Read the model definition and answer for the solid it produces. Units are mm, in the model's axes. Coordinates: 2 decimals unless noted, no trailing zeros. Order: outer loops, then holes, each group sorted by start corner. A loop starts at its lowest first (then second) coordinate and runs counter-clockwise, first axis right, second up. Notation, with made-up numbers: M 7,-8.5 L 29,-8.5 A6 ccw 29,-0.5 Z; hole C 35.25,61.25 d10. An arc over 180 degrees is marked long. Use a Markdown table: item, result. Add a question column.
1) Find section B-B on x = 131.15. Write down the section's boundary in (y, z), plus the area to 3 significant figures.
2) Find section D-D on x = 30.5. Write down the section's boundary in (y, z), plus the area to 3 significant figures.
3) Find section C-C on y = 2. Count the separate pieces of the cut face and the enclosed holes in it, plus the area to 3 significant figures.
4) Find the intervals of material crossed by probe 1 along X at (y, z) = (4.5, -50); probe 2 along Z at (x, y) = (119, 4.25); probe 3 along Z at (x, y) = (131.15, 4.5), in increasing order. Write a range as [from, to].
5) This flat-tipped pin is pushed along its axis until it touches: pin 1 Ø2.5 at (x, z) = (8.85, -50) entering from -Y. Where does it stop, or does it pass through?
6) Find section A-A on x = 68. Write down the section's boundary in (y, z), plus the area to 3 significant figures.
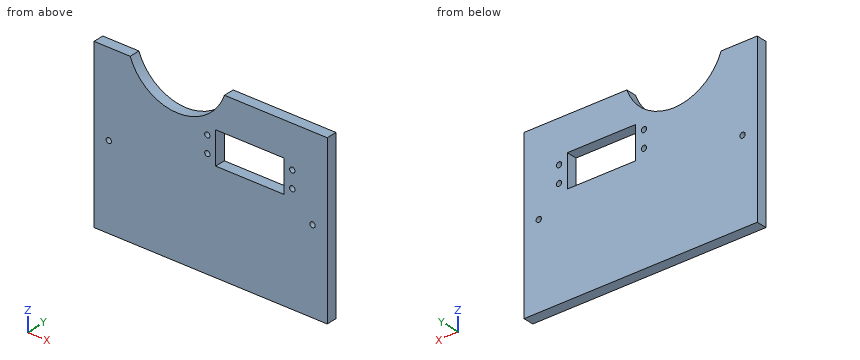
from build123d import *

# Parameters (mm, degrees)
SKETCH1_W           = 140
SKETCH1_H           = 100
BOSS_EXTRUDE1_DEPTH = 6.35
SKETCH2_W           = 41
SKETCH2_H           = 19.5
CUT_EXTRUDE1_DEPTH  = 10
SKETCH3_R           = 30
CUT_EXTRUDE2_DEPTH  = 10
SKETCH4_R           = 1.5875
CUT_EXTRUDE3_DEPTH  = 10


with BuildPart() as part:
    # Sketch1 → Boss-Extrude1 (new body)
    with BuildSketch(Plane(origin=(0, 0, 0), x_dir=(1, 0, 0), z_dir=(0, 1, 0))):
        with Locations((70, 50)):
            Rectangle(SKETCH1_W, SKETCH1_H)
    extrude(amount=BOSS_EXTRUDE1_DEPTH)

    # Sketch2 → Cut-Extrude1 (cut)
    with BuildSketch(Plane(origin=(0, 6.35, 0), x_dir=(1, 0, 0), z_dir=(0, 1, 0))):
        with Locations((93.5, 30.25)):
            Rectangle(SKETCH2_W, SKETCH2_H)
    extrude(amount=-CUT_EXTRUDE1_DEPTH, mode=Mode.SUBTRACT)

    # Sketch3 → Cut-Extrude2 (cut)
    with BuildSketch(Plane(origin=(0, 6.35, 0), x_dir=(1, 0, 0), z_dir=(0, 1, 0))):
        with Locations((50, -10)):
            Circle(SKETCH3_R)
    extrude(amount=-CUT_EXTRUDE2_DEPTH, mode=Mode.SUBTRACT)

    # Sketch4 → Cut-Extrude3 (cut)
    with BuildSketch(Plane(origin=(0, 6.35, 0), x_dir=(1, 0, 0), z_dir=(0, 1, 0))):
        with Locations(Location((131.15, 50, 0), (0, 0, 270))):
            Circle(SKETCH4_R)
        with Locations(Location((8.85, 50, 0), (0, 0, 270))):
            Circle(SKETCH4_R)
        with Locations(Location((68, 25.125, 0), (0, 0, 270))):
            Circle(SKETCH4_R)
        with Locations(Location((119, 35.125, 0), (0, 0, 270))):
            Circle(SKETCH4_R)
        with Locations(Location((68, 35.125, 0), (0, 0, 270))):
            Circle(SKETCH4_R)
        with Locations(Location((119, 25.125, 0), (0, 0, 270))):
            Circle(SKETCH4_R)
    extrude(amount=-CUT_EXTRUDE3_DEPTH, mode=Mode.SUBTRACT)


solid = part.part
Check result:
| question | item | result |
|---|---|---|
| 1 | outline | M 0,-100 L 6.35,-100 L 6.35,-51.59 L 0,-51.59 Z; M 0,-48.41 L 6.35,-48.41 L 6.35,0 L 0,0 Z |
| 1 | area | 615 mm2 |
| 2 | outline | M 0,-100 L 6.35,-100 L 6.35,-12.8 L 0,-12.8 Z |
| 2 | area | 554 mm2 |
| 3 | separate pieces | 1 |
| 3 | enclosed holes | 7 |
| 3 | area | 12,300 mm2 |
| 4 | probe 1 | x = [0, 7.26], [10.44, 129.56], [132.74, 140] |
| 4 | probe 2 | z = [-100, -36.71], [-33.54, -26.71], [-23.54, 0] |
| 4 | probe 3 | z = [-100, -51.59], [-48.41, 0] |
| 5 | pin 1 | passes through |
| 6 | outline | M 0,-100 L 6.35,-100 L 6.35,-36.71 L 0,-36.71 Z; M 0,-33.54 L 6.35,-33.54 L 6.35,-26.71 L 0,-26.71 Z; M 0,-23.54 L 6.35,-23.54 L 6.35,-14 L 0,-14 Z |
| 6 | area | 506 mm2 |
